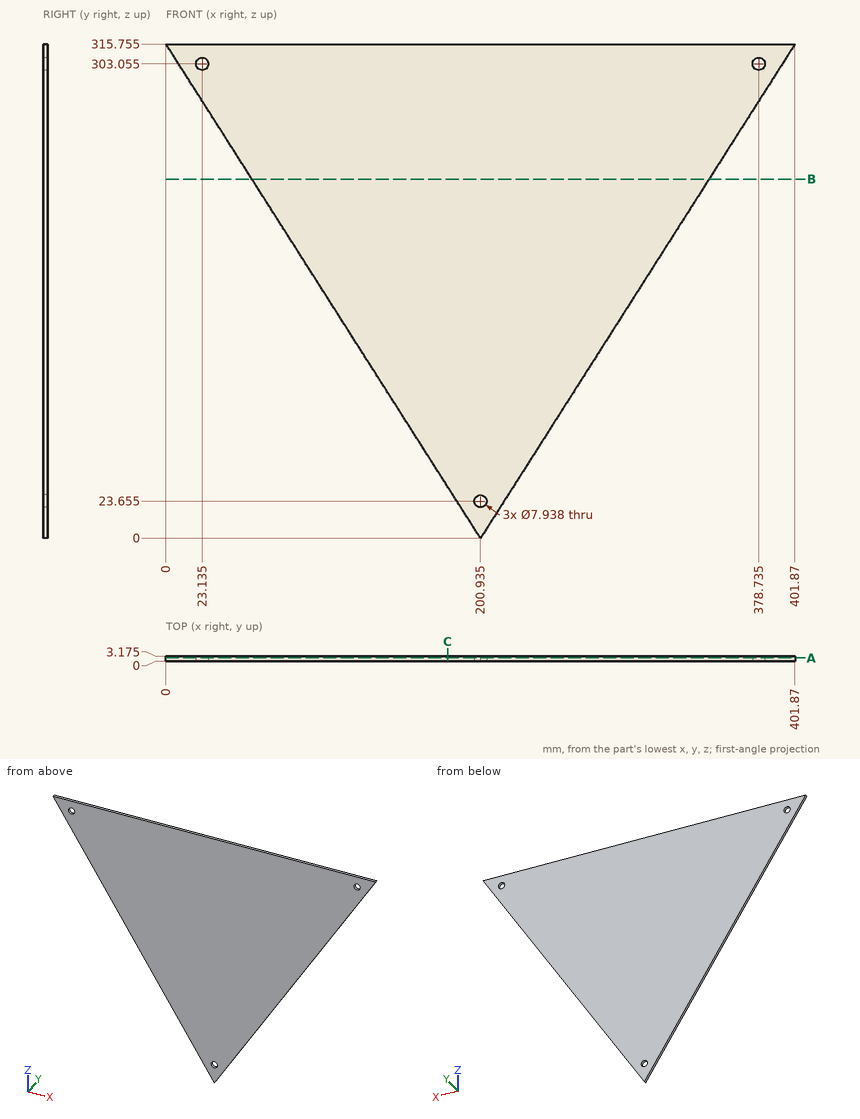
Part print with two shaded views. Sizes in mm from the minimum x, y, z corner. Coordinates: 2 decimals unless noted, no trailing zeros. Write each loop counter-clockwise with the first axis right and the second up, starting at its lowest first coordinate (ties: lowest second). Pieces come first, ordered by that corner, then holes. Notation, with made-up numbers: M 34,44 L 55,44 A23 cw 55,74 Z; hole C -28,48 d11. An arc over 180 degrees is marked long. Return JSON: item names as keys, results as strings.
Item 1: Slice it at B-B, the plane z = 229.5. Write the cut outline in (x, y) (1 decimal).
Findings below:
{"outline": "M 54.9,0 L 347,0 L 347,3.2 L 54.9,3.2 Z"}
Item 2: Drop flat-ended pins along their axis: pin 1 Ø7 at (x, z) = (200.94, 23.66) entering from -Y; pin 2 Ø1.5 at (x, y) = (118, 1.5) entering from -Z. Give the stop position or say it passes through.
Findings below:
{"pin 1": "passes through", "pin 2": "stops at z = 129.15"}
Item 3: Slice it at C-C, the plane x = 180. Write the cut outline in (y, z) (1 decimal).
Findings below:
{"outline": "M 0,32.9 L 3.2,32.9 L 3.2,315.8 L 0,315.8 Z"}
Item 4: Slice it at A-A, the plane y = 2.2. Write the cut outline in (x, z) (1 decimal), and give its area (3 significant figures).
Findings below:
{"outline": "M 0,315.8 L 200.9,0 L 401.9,315.8 Z; hole C 23.1,303.1 d7.9; hole C 200.9,23.7 d7.9; hole C 378.7,303.1 d7.9", "area": "63,300 mm2"}
Item 5: Probe line 1 (Z direction, x = 21, y = 2.45) (1 decimal); line 2 (Z direction, x = 347.5, y = 1.1) (1 decimal); line 3 (Z direction, x = 352.5, y = 2.65) (1 decimal). List the from-to ranges inside material, lowest first. Write a range as from..to.
Findings below:
{"line 1": "z = 282.8..299.7, 306.4..315.8", "line 2": "z = 230.3..315.8", "line 3": "z = 238.2..315.8"}
